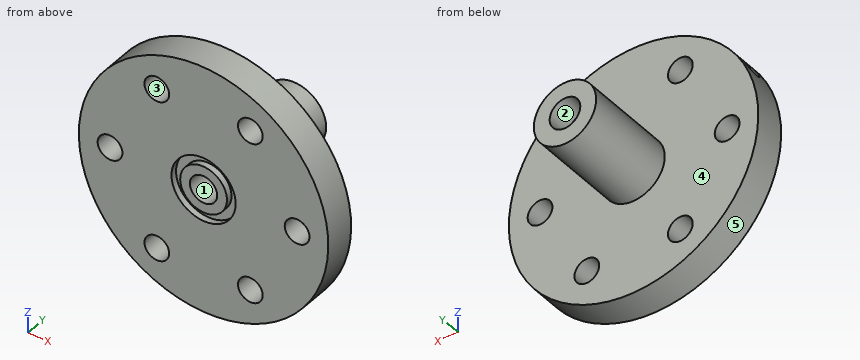
```python
from build123d import *

# Parameters (mm, degrees)
F_3_8_CLEARANCE_HOLE1_D              = 10.0838
CIRPATTERN1_COUNT                    = 6
F_1_32_0_03125_DIAMETER_HOLE1_REACH  = 133.807
F_1_32_0_03125_DIAMETER_HOLE1_BORE_R = 0.396875
F_1_4_0_25_DIAMETER_HOLE1_D          = 6.35
F_1_4_0_25_DIAMETER_HOLE1_DEPTH      = 12.7
F_1_4_0_25_DIAMETER_HOLE1_TIP        = 1.907732465


with BuildPart() as part:
    # Sketch1 → Revolve1 (revolve)
    with BuildSketch(Plane.XY, mode=Mode.PRIVATE) as revolve1_sk:
        Polygon((0, 0), (-12.7, 0), (-12.7, -38.1), (-50.8, -38.1), (-50.8, -50.8), (-13.081, -50.8), (-13.081, -48.26), (-9.525, -48.26), (-9.525, -50.8), (0, -50.8), align=None)
    revolve(revolve1_sk.sketch.rotate(Axis((0, -50.8, 0), (0, 1, 0)), 270), axis=Axis((0, -50.8, 0), (0, 1, 0)))

    # Sketch4 → 1/4 NPT Tapped Hole1 (revolve, cut)
    with BuildSketch(Plane(origin=(0, 0, 0), x_dir=(0, 0, 1), z_dir=(1, 0, 0))):
        Polygon((0, 0), (0, 50.8), (5.5626, 50.8), (5.5626, 9.906), (5.943685794, 9.906), (6.2402847, 0), align=None)
    revolve(axis=Axis((0, 6.35, 0), (0, -1, 0)), mode=Mode.SUBTRACT)

    # 3/8 Clearance Hole1 (through all)
    with Locations(Plane(origin=(0, -38.1, 0), x_dir=(1, 0, 0), z_dir=(0, 1, 0))):
        with Locations((38.1, 0)):
            f_3_8_clearance_hole1 = Hole(F_3_8_CLEARANCE_HOLE1_D / 2)

    # CirPattern1: 3/8 Clearance Hole1 ×6 about axis
    cirpattern1_axis = Axis((0, 0, 0), (0, 1, 0))
    for i in range(1, CIRPATTERN1_COUNT):
        add(f_3_8_clearance_hole1.rotate(cirpattern1_axis, i * 360 / CIRPATTERN1_COUNT), mode=Mode.SUBTRACT)

    # 1/32 (0.03125) Diameter Hole1 bore → 1/32 (0.03125) Diameter Hole1 (cut, up to next)
    with BuildSketch(Plane(origin=(-43.994090512, 0, 25.4), x_dir=(0, -1, 0), z_dir=(-0.8660254037844398, 0, 0.499999999999998)), mode=Mode.PRIVATE) as f_1_32_0_03125_diameter_hole1_sk1:
        with Locations((44.45, 0)):
            Circle(F_1_32_0_03125_DIAMETER_HOLE1_BORE_R)
    f_1_32_0_03125_diameter_hole1_tool1 = extrude(f_1_32_0_03125_diameter_hole1_sk1.sketch, amount=-F_1_32_0_03125_DIAMETER_HOLE1_REACH, mode=Mode.PRIVATE) & part.part
    add(f_1_32_0_03125_diameter_hole1_tool1.solids().sort_by_distance((-43.994091, -44.45, 25.4))[0], mode=Mode.SUBTRACT)

    # 1/4 (0.25) Diameter Hole1
    with Locations(Plane(origin=(-43.994090512, 0, 25.4), x_dir=(0, -1, 0), z_dir=(-0.8660254037844398, 0, 0.499999999999998))):
        with Locations((44.45, 0)):
            Hole(F_1_4_0_25_DIAMETER_HOLE1_D / 2, depth=F_1_4_0_25_DIAMETER_HOLE1_DEPTH)
            with Locations((0, 0, -(F_1_4_0_25_DIAMETER_HOLE1_DEPTH + F_1_4_0_25_DIAMETER_HOLE1_TIP / 2))):  # 118° drill point
                Cone(0, F_1_4_0_25_DIAMETER_HOLE1_D / 2, F_1_4_0_25_DIAMETER_HOLE1_TIP, mode=Mode.SUBTRACT)


solid = part.part
```
Check sheet for the modelled part. Datum: model origin and axes. Units: mm. Face numbers are marked on the shaded views. A direction names the side the tool comes from. Round coordinates to 2 decimals unless told otherwise and drop trailing zeros. Order: outer loops, then holes, each group sorted by start corner. A loop starts at its lowest first (then second) coordinate and runs counter-clockwise, first axis right, second up. Notation, with made-up numbers: (3.5, 63) - (53.5, 63) arc R38 ccw to (53.5, 101) - close; hole circle Ø1 at (25.25, 11). An arc over 180 degrees is marked (long way). Answer as CSV lines item,"result". Start each with the question number.
1) Tool access check on the marked faces 1 and 2. Record the directions out of +Z, -Z, +X, -X, +Y, -Y that give a thin tool (end or side, any length) a straight path to the whole face; none if there is none.
2) Scan lines: probe 1 along X at (y, z) = (-12, 0); probe 2 along Z at (x, y) = (19.05, -42); probe 3 along X at (y, z) = (-48.5, 29). Record each from-to range of solid material in increasing order.
3) Section check C-C (z = 30.5). Record the cut outline in (x, y) (3 decimals).
4) Section check B-B (z = 0). Give the number of separate pieces and of enclosed holes in the cut face, then the cut area to 3 significant figures.
5) Draft check along Z on the marked faces 3, 4 and 5. Enter one of: +Z half, -Z half, draft (parallel to the pull), parting line (faces both ways), or undercut.
6) Depth check by flat-ended pin: pin 1 (12 mm diameter, centred on x = 1, z = 22.5, fed in from +Y); pin 2 (1.5 mm diameter, centred on x = 10, y = -19.5, fed in from +Z); pin 3 (1 mm diameter, centred on x = -11.5, y = -40.5, fed in from +Z). Enter the tip coordinate at first touch or a pass-through.
7) Section check A-A (x = 0). Record the cut outline in (y, z) (3 decimals), then the cut area to 3 significant figures.
Determined:
1,face 1,"+Y, -Y"
1,face 2,"+Y"
2,probe 1,"-12.7 to -5.56, 5.56 to 12.7"
2,probe 2,"-47.09 to -38.04, -27.95 to 27.95, 38.04 to 47.09"
2,probe 3,"-41.71 to -22.13, -15.97 to 15.97, 22.13 to 41.71"
3,outline,"(-40.625, -50.8) - (-23.431, -50.8) - (-23.431, -38.1) - (-40.625, -38.1) - close; (-14.669, -50.8) - (14.669, -50.8) - (14.669, -38.1) - (-14.669, -38.1) - close; (23.431, -50.8) - (40.625, -50.8) - (40.625, -38.1) - (23.431, -38.1) - close"
4,separate pieces,"4"
4,enclosed holes,"0"
4,area,"1,410 mm^2"
5,face 3,"undercut"
5,face 4,"draft"
5,face 5,"parting line"
6,pin 1,"y = -38.1"
6,pin 2,"z = 8.7"
6,pin 3,"z = 49.59"
7,outline,"(-50.8, -50.8) - (-38.1, -50.8) - (-38.1, -12.7) - (0, -12.7) - (0, -6.24) - (-9.906, -5.944) - (-9.906, -5.563) - (-50.8, -5.563) - (-50.8, -9.525) - (-48.26, -9.525) - (-48.26, -13.081) - (-50.8, -13.081) - close; (-50.8, 5.563) - (-9.906, 5.563) - (-9.906, 5.944) - (0, 6.24) - (0, 12.7) - (-38.1, 12.7) - (-38.1, 50.8) - (-50.8, 50.8) - (-50.8, 13.081) - (-48.26, 13.081) - (-48.26, 9.525) - (-50.8, 9.525) - close"
7,area,"1,660 mm^2"
